Geometry check sheet. Reference: drawing and pictorial views, mm from the part's lowest x, y, z. A direction names the side the tool comes from. Give positions to 0.01 mm unless a question says otherwise; leave off trailing zeros. Order: outer loops, then holes, each group sorted by start corner. A loop starts at its lowest first (then second) coordinate and runs counter-clockwise, first axis right, second up.
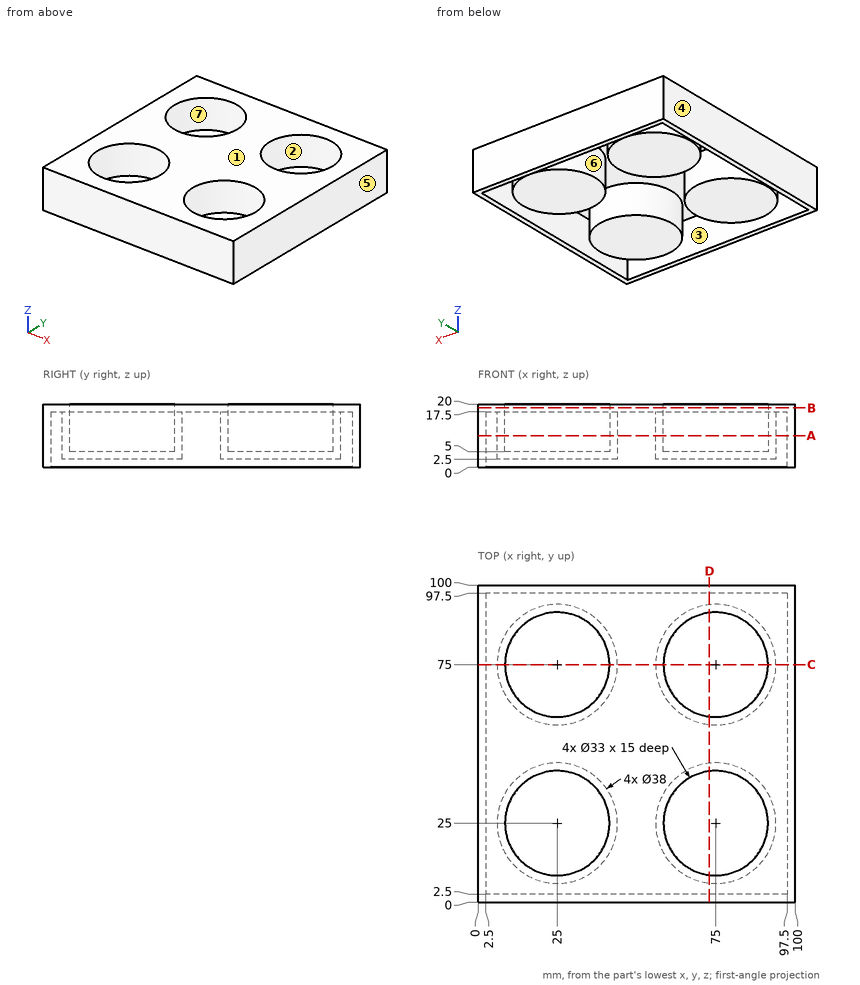
(1) Cross-section at D-D on x = 73. Enter the section's corners in (y, z), then the cut area to 3 significant figures.
Response values:
outline: (0, 0) - (2.5, 0) - (2.5, 17.5) - (6.11, 17.5) - (6.11, 2.5) - (43.89, 2.5) - (43.89, 17.5) - (56.11, 17.5) - (56.11, 2.5) - (93.89, 2.5) - (93.89, 17.5) - (97.5, 17.5) - (97.5, 0) - (100, 0) - (100, 20) - (91.38, 20) - (91.38, 5) - (58.62, 5) - (58.62, 20) - (41.38, 20) - (41.38, 5) - (8.62, 5) - (8.62, 20) - (0, 20) - close
area: 488 mm2
(2) Cross-section at B-B on z = 18.75. Enter the section's corners in (x, y), then the cut area to 3 significant figures.
Response values:
outline: (0, 0) - (100, 0) - (100, 100) - (0, 100) - close; hole circle Ø33 at (25, 25); hole circle Ø33 at (25, 75); hole circle Ø33 at (75, 25); hole circle Ø33 at (75, 75)
area: 6,580 mm2
(3) Set-up check for the marked faces 5, 6 and 7: record each of +Z, -Z, +X, -X, +Y, -Y from which the full face is reachable in a straight line by a thin tool's end or side.
Response values:
face 5: +Z, -Z, +X, +Y, -Y
face 6: -Z
face 7: +Z
(4) Cross-section at C-C on y = 75. Enter the section's corners in (x, z).
Response values:
outline: (0, 0) - (2.5, 0) - (2.5, 17.5) - (6, 17.5) - (6, 2.5) - (44, 2.5) - (44, 17.5) - (56, 17.5) - (56, 2.5) - (94, 2.5) - (94, 17.5) - (97.5, 17.5) - (97.5, 0) - (100, 0) - (100, 20) - (91.5, 20) - (91.5, 5) - (58.5, 5) - (58.5, 20) - (41.5, 20) - (41.5, 5) - (8.5, 5) - (8.5, 20) - (0, 20) - close
(5) Gauge pin test, flat ends, axial feed: pin 1 Ø11.5 at (x, y) = (17.5, 76) entering from -Z; pin 2 Ø6 at (x, y) = (37, 22.5) entering from +Z; pin 3 Ø2 at (x, y) = (51, 26.5) entering from -Z. Record the tip position at first contact, or that the pin passes through.
Response values:
pin 1: stops at z = 2.5
pin 2: stops at z = 5
pin 3: stops at z = 17.5
(6) Cross-section at A-A on z = 10. Count the separate pieces of the cut face and the enclosed holes in it, then the cut area to 3 significant figures.
Response values:
separate pieces: 5
enclosed holes: 5
area: 2,090 mm2
(7) Material ranges on L1, parallel to Y at x = 25, z = 12.75; L2, parallel to X at y = 77.5, z = 13; L3, parallel to X at y = 86.5, z = 7, recorded low to high.
Response values:
L1: y = 0 to 2.5, 6 to 8.5, 41.5 to 44, 56 to 58.5, 91.5 to 94, 97.5 to 100
L2: x = 0 to 2.5, 6.17 to 8.69, 41.31 to 43.83, 56.17 to 58.69, 91.31 to 93.83, 97.5 to 100
L3: x = 0 to 2.5, 9.88 to 13.17, 36.83 to 40.12, 59.88 to 63.17, 86.83 to 90.12, 97.5 to 100
(8) Release check for a two-part mould opening along X. For the marked faces 1, 2, 3 and 4 record: released by +X, released by -X, zero draft, split by the parting line, or undercut.
Response values:
face 1: zero draft
face 2: undercut
face 3: undercut
face 4: released by -X
